Autodesk Inventor part; units mm, degrees
ref_plane "YZ Plane" through (0, 0, 0) normal (1, 0, 0) x (0, 1, 0)
ref_plane "XZ Plane" through (0, 0, 0) normal (0, 1, 0) x (-1, 0, 0)
ref_plane "XY Plane" through (0, 0, 0) normal (0, 0, 1) x (1, 0, 0)
sketch "main" plane through (0, 0, 0) normal (0, 0, 1) x (1, 0, 0)
  circle A0 centre (-24.2926, 27.4457) radius 2.1844
  circle A1 centre (-24.2926, -23.3543) radius 2.1844
  circle A2 centre (26.5074, 27.4457) radius 2.1844
  arc A3 (-30.6426, -23.3543) -> (-19.8025, -27.8444) centre (-24.2926, -23.3543) ccw
  arc A4 (30.9975, 22.9556) -> (26.5074, 33.7957) centre (26.5074, 27.4457) ccw
  arc A5 (-24.2926, 33.7957) -> (-30.6426, 27.4457) centre (-24.2926, 27.4457) ccw
  line L0 (-30.6426, -23.3543) -> (-30.6426, 27.4457)
  line L1 (-24.2926, 33.7957) -> (26.5074, 33.7957)
  line L2 (30.9975, 22.9556) -> (-19.8025, -27.8444)
  line L3 (-16.3551, -4.1915) -> (7.3446, 19.5082)
  line L4 (7.3446, 19.5082) -> (-16.3551, 19.5082)
  line L5 (-16.3551, 19.5082) -> (-16.3551, -4.1915)
  point P0 (-7.9432, 11.0963)
  dimension "d0" = 12.7
  dimension "d1" = 12.7
  dimension "d2" = 12.7
  dimension "d3" = 14.2875
sketch "Sketch1" plane through (0, 0, 0) normal (0, 1, 0) x (-1, 0, 0)
  circle A0 centre (0, 0) radius 2.1844
  circle A1 centre (0, -50.8) radius 2.1844
  circle A2 centre (50.8, 0) radius 2.1844
  arc A3 (-6.35, -50.8) -> (4.4901, -55.2901) centre (0, -50.8) ccw
  arc A4 (55.2901, -4.4901) -> (50.8, 6.35) centre (50.8, 0) ccw
  arc A5 (0, 6.35) -> (-6.35, 0) centre (0, 0) ccw
  line L0 (-6.35, -50.8) -> (-6.35, 0)
  line L1 (0, 6.35) -> (50.8, 6.35)
  line L2 (55.2901, -4.4901) -> (4.4901, -55.2901)
  line L3 (7.9375, -31.6372) -> (31.6372, -7.9375)
  line L4 (31.6372, -7.9375) -> (7.9375, -7.9375)
  line L5 (7.9375, -7.9375) -> (7.9375, -31.6372)
extrude "Extrusion1" add sketch "Sketch1" along normal blind 1.5875
properties part number "Triangle Gusset" material "Acetal Resin, White"
The model under review builds one solid part; all positions refer to its coordinate system, in mm. A direction names the side the tool comes from. Give positions to 0.01 mm unless a question says otherwise; leave off trailing zeros. Loops run counter-clockwise (first coordinate to the right, second up) from the corner with the lowest first, then second, coordinate; pieces in that order, holes last. Notation, with made-up numbers: (9, -15) -> (50, -15) arc R8 cw to (50, -10) -> close; hole circle Ø6 at (-19.75, 19). An arc over 180 degrees is marked (long way). Use CSV: the item, a comma, the result in double quotes.
1. Consider section D-D, the plane z = -44.5. Write out the cut boundary in (x, y), then the cut area to 3 significant figures.
Result:
outline,"(-15.28, 0) -> (6.35, 0) -> (6.35, 1.59) -> (-15.28, 1.59) -> close"
area,"34.3 mm²"
2. Machinability: for faces 5 (the face through (-56.626, 0.783, 2.526)), 6 (the face through (-20, 1, -7.938)), which of the approach directions +Z, -Z, +X, -X, +Y, -Y give a long, thin tool a straight path to every point of the face, cutting with its end or side? Answer none if there is none.
Result:
face 5,"-X, +Y, -Y"
face 6,"+Y, -Y"
3. The part is to be moulded in two halves that separate along Z. For faces 1 (the face through (-25, 0, -18)), 2 (the face through (-25, 1, 6.35)), 3 (the face through (-1.174, 0.783, -52.642)), 4 (the face through (2.333, 0.783, -56.706)), say which applies: +Z half, -Z half, draft (parallel to the pull), parting line (faces both ways), or undercut.
Result:
face 1,"draft"
face 2,"+Z half"
face 3,"undercut"
face 4,"-Z half"
4. Consider section C-C, the plane x = -30.5. Write out the cut boundary in (y, z), then the cut area to 3 significant figures.
Result:
outline,"(0, -29.28) -> (1.59, -29.28) -> (1.59, -9.07) -> (0, -9.07) -> close; (0, -7.94) -> (1.59, -7.94) -> (1.59, 6.35) -> (0, 6.35) -> close"
area,"54.8 mm²"
5. To check wall thickness, follow probe 1 along Z at (x, y) = (0, 1.15); probe 2 along X at (y, z) = (0.9, -13); probe 3 along X at (y, z) = (0.3, -52). State the ranges of each line that lie inside material, in increasing order. Write a range as from..to.
Result:
probe 1,"z = -57.15..-52.98, -48.62..-2.18, 2.18..6.35"
probe 2,"x = -46.78..-26.57, -7.94..6.35"
probe 3,"x = -7.78..-1.83, 1.83..6.24"
6. Consider section A-A, the plane y = 0.55. Write out the cut boundary in (x, z).
Result:
outline,"(-55.29, -4.49) -> (-4.49, -55.29) arc R6.35 ccw to (6.35, -50.8) -> (6.35, 0) arc R6.35 ccw to (0, 6.35) -> (-50.8, 6.35) arc R6.35 ccw to start; hole circle Ø4.37 at (-50.8, 0); hole (-31.64, -7.94) -> (-7.94, -31.64) -> (-7.94, -7.94) -> close; hole circle Ø4.37 at (0, -50.8); hole circle Ø4.37 at (0, 0)"
7. For P1, Ø3.5, axis at x = 0, z = 0, coming from the -Y side; P2, Ø5.5, axis at x = 0, z = -50.8, coming from the +Y side; P3, Ø0.8, axis at y = 0.5, z = -20, coming from the -X side, all flat-tipped, find the tip position at first contact; note any pin that passes through.
Result:
P1,"passes through"
P2,"stops at y = 1.59"
P3,"stops at x = -40.18"
8. Consider section B-B, the plane z = -17. Write out the cut boundary in (x, y), then the cut area to 3 significant figures.
Result:
outline,"(-42.78, 0) -> (-22.57, 0) -> (-22.57, 1.59) -> (-42.78, 1.59) -> close; (-7.94, 0) -> (6.35, 0) -> (6.35, 1.59) -> (-7.94, 1.59) -> close"
area,"54.8 mm²"
